Design review of the part built by this model. Coordinates are the model's own, in mm. A direction names the side the tool comes from. Give positions to 0.01 mm unless a question says otherwise; leave off trailing zeros. Order: outer loops, then holes, each group sorted by start corner. A loop starts at its lowest first (then second) coordinate and runs counter-clockwise, first axis right, second up.
```python
from build123d import *

# Parameters (mm, degrees)
BOSS_EXTRUDE1_DEPTH = 50
SKETCH4_OUTSIDE_W   = 144.624
SKETCH4_OUTSIDE_H   = 79.42
SKETCH4_OUTSIDE_R   = 8.345
CUT_EXTRUDE1_DEPTH  = 99.876606464
SKETCH5_R           = 10
BOSS_EXTRUDE2_DEPTH = 40


with BuildPart() as part:
    # Sketch3 → Boss-Extrude1 (new body)
    with BuildSketch(Plane(origin=(0, 0, 0), x_dir=(1, 0, 0), z_dir=(0, 1, 0))):
        with BuildLine():
            Line((-12.5, 0), (-12.5, 50))
            Line((-12.5, 50), (-27.5, 50))
            Line((-27.5, 50), (-27.5, 0))
            ThreePointArc((-27.5, 0), (-23.00815073, -15.062370331), (-11, -25.204166322))
            Line((-11, -25.204166322), (-11, -65.204166322))
            Line((-11, -65.204166322), (11, -65.204166322))
            Line((11, -65.204166322), (11, -25.204166322))
            ThreePointArc((11, -25.204166322), (23.00815073, -15.062370331), (27.5, 0))
            Line((27.5, 0), (27.5, 37.66))
            Line((27.5, 37.66), (12.5, 37.66))
            Line((12.5, 37.66), (12.5, 0))
            ThreePointArc((12.5, 0), (0, -12.5), (-12.5, 0))
        make_face()
    extrude(amount=BOSS_EXTRUDE1_DEPTH)

    # Sketch4 outside → Cut-Extrude1 (cut, through all)
    # profile 1 of 2: a face of its own
    with BuildSketch(Plane(origin=(27.5, 0, 0), x_dir=(0, 0, -1), z_dir=(1, 0, 0))):
        with Locations((-7.602, 25)):
            Rectangle(SKETCH4_OUTSIDE_W, SKETCH4_OUTSIDE_H)
        with BuildLine():
            Line((-9.789944321, 14), (-65.204166322, 14))
            Line((-65.204166322, 14), (-65.204166322, 36))
            Line((-65.204166322, 36), (-9.789944321, 36))
            ThreePointArc((-9.789944321, 36), (37.66, 25), (-9.789944321, 14))
        make_face(mode=Mode.SUBTRACT)
    # profile 2 of 2: a face of its own
    with BuildSketch(Plane(origin=(27.5, 0, 0), x_dir=(0, 0, -1), z_dir=(1, 0, 0))):
        with Locations((12.66, 25)):
            Circle(SKETCH4_OUTSIDE_R)
    extrude(amount=-CUT_EXTRUDE1_DEPTH, mode=Mode.SUBTRACT)

    # Sketch5 → Boss-Extrude2 (add)
    with BuildSketch(Plane.XY.offset(65.204166322)):
        with Locations((0, 25)):
            Circle(SKETCH5_R)
    extrude(amount=BOSS_EXTRUDE2_DEPTH)


solid = part.part
```
1. For pin 1 (8 mm diameter, centred on x = -18.5, y = 10.5, fed in from -Z); pin 2 (6.5 mm diameter, centred on y = 24.5, z = 52, fed in from -X); pin 3 (6 mm diameter, centred on x = -5, z = 23, fed in from -Y); pin 4 (15 mm diameter, centred on y = 25, z = -12.66, fed in from +X), all flat-tipped, find the tip position at first contact; note any pin that passes through.
Recorded:
pin 1: stops at z = -35.35
pin 2: stops at x = -11
pin 3: stops at y = 14
pin 4: passes through
2. For line 1 along Y through (x, z) = (-16.25, -12.66) (3 decimals); line 2 along X through (y, z) = (14.5, -20); line 3 along Z through (x, y) = (20.5, 18), list the stretches that pass through material, from the lowest coordinate up.
Recorded:
line 1: y = 0 to 16.655, 33.345 to 50
line 2: x = -27.5 to -12.5, 12.5 to 27.5
line 3: z = -36.66 to -17.2, -8.12 to 18.33
3. Take a section at D-D (x = -22). State the section outline as (y, z) points (3 decimals).
Recorded:
outline: (14, 9.79) arc R25 ccw (long way) to (36, 9.79) - (36, 16.5) - (14, 16.5) - close; hole circle Ø16.69 at (25, -12.66)
4. Take a section at C-C (y = 45). State the section outline as (x, z) points, then the cut area to 3 significant figures.
Recorded:
outline: (-27.5, -27.66) - (-12.5, -27.66) - (-12.5, 0) arc R12.5 cw to (-12.28, 2.34) - (-27.4, 2.34) arc R27.5 ccw to (-27.5, 0) - close; (12.28, 2.34) arc R12.5 cw to (12.5, 0) - (12.5, -27.66) - (27.5, -27.66) - (27.5, 0) arc R27.5 ccw to (27.4, 2.34) - close
area: 900 mm2
5. Take a section at A-A (z = -12.66). State the section outline as (x, y) points (3 decimals), then the cut area to 3 significant figures.
Recorded:
outline: (-27.5, 0) - (-12.5, 0) - (-12.5, 16.655) - (-27.5, 16.655) - close; (-27.5, 33.345) - (-12.5, 33.345) - (-12.5, 50) - (-27.5, 50) - close; (12.5, 0) - (27.5, 0) - (27.5, 16.655) - (12.5, 16.655) - close; (12.5, 33.345) - (27.5, 33.345) - (27.5, 50) - (12.5, 50) - close
area: 999 mm2
6. Take a section at B-B (x = 0). State the section outline as (y, z) points, then the cut area to 3 significant figures.
Recorded:
outline: (14, 12.5) - (36, 12.5) - (36, 65.2) - (35, 65.2) - (35, 105.2) - (15, 105.2) - (15, 65.2) - (14, 65.2) - close
area: 1,960 mm2
7. Machinability: for faces 1 (the face through (-11, 25, 45)), 2 (the face through (11, 25, 45)), 3 (the face through (0, 14, 31)), which of the approach directions +Z, -Z, +X, -X, +Y, -Y give a long, thin tool a straight path to every point of the face, cutting with its end or side? Answer none if there is none.
Recorded:
face 1: +Z, -X, +Y, -Y
face 2: +Z, +X, +Y, -Y
face 3: +Z, +X, -X, -Y
8. Draft analysis for pull direction Z (two halves, no side actions). For faces 4 (the face through (20.105, 16.853, -10.851)), 5 (the face through (22.885, 24.698, 15.249)), 6 (the face through (-19.69, 25.94, -37.642)), state which applies: pulls with the +Z half, pulls with the -Z half, needs draft (parallel to the pull), parting line crosses it, or undercut.
Recorded:
face 4: undercut
face 5: pulls with the +Z half
face 6: parting line crosses it
